Build history of the part. All positions in model axes, mm. A direction names the side the tool comes from. Give positions to 0.01 mm unless a question says otherwise; leave off trailing zeros. Write each loop counter-clockwise with the first axis right and the second up, starting at its lowest first coordinate (ties: lowest second). Pieces come first, ordered by that corner, then holes. Notation, with made-up numbers: (23.5, 34) -> (44.5, 34) arc R18 cw to (44.5, 51) -> close; hole circle Ø2 at (49.5, 9.5). An arc over 180 degrees is marked (long way). Put each result on its own line as item: value. Start each with the question number.
Item 1: Slice it at C-C, the plane x = 13. List the corners of the cut face in (y, z).
Item 2: Flat gauge pins, fed straight in: pin 1 Ø0.5 at (x, z) = (-16.5, 4.5) entering from -Y; pin 2 Ø3 at (y, z) = (-13.5, 5) entering from -X; pin 3 Ø0.7 at (x, z) = (-16.5, 3) entering from +Y; pin 4 Ø1.8 at (x, y) = (13, -5) entering from +Z. Where does each tip first touch, or does it go through?
Item 3: Slice it at B-B, the plane z = 5.5. List the corners of the cut face in (x, y).
Item 4: Tool access for faces 5 (the flat face through (0, 0, 4.2)), 6 (the flat face through (15.321, -9.837, 1.232)), 7 (the flat face through (-16.45, 7.76, 8.73)): list every direction of +Z, -Z, +X, -X, +Y, -Y with a clear straight run to the whole face (end or side of a thin tool).
Item 5: Slice it at A-A, the plane y = -5. List the corners of the cut face in (x, z).
Item 6: Drill centre lines: line 1 along X through (y, z) = (-5, 6.25); line 2 along Y through (x, z) = (-13, 5.5); line 3 along Z through (x, y) = (-16, -9.5). Where is each one in solid material? Low to high.
Item 7: Slice it at D-D, the plane x = 5. List the corners of the cut face in (y, z).
Item 8: Two-plate mould, pull along Z, no slides. Class faces 1 (the cylindrical face through (0.037, 3.795, 2.071)), 2 (the flat face through (0, 0, 10)), 3 (the flat face through (-2, -18, 2.5)), 4 (the flat face through (0, -4, 0)): pulls with the +Z half, pulls with the -Z half, needs draft (parallel to the pull), parting line crosses it, or undercut.
```python
from build123d import *

# Parameters (mm, degrees)
CROQUIS1_R                   = 17.7
SALIENTE_EXTRUIR1_DEPTH      = 10
ENVOLVER1_SECTION_W          = 1
ENVOLVER1_SECTION_H          = 2.5
ENVOLVER1_ANGLE              = 122.036773313
ENVOLVER1_SECTOR_2_SECTION_W = 1
ENVOLVER1_SECTOR_2_SECTION_H = 2.5
ENVOLVER1_SECTOR_2_ANGLE     = 122.036773313
SIMETR_A1_DEPTH              = 2.5
SIMETR_A1_START              = 7.5
SIMETR_A1_2_DEPTH            = 2.5
CAVIDAD1_DEPTH               = 4.2
SALIENTE_EXTRUIR2_START      = 4.2
SALIENTE_EXTRUIR2_DEPTH      = 4.2
CROQUIS6_R                   = 1.5
CORTAR_EXTRUIR1_DEPTH        = 10
CROQUIS8_W                   = 1.5
CROQUIS8_H                   = 1
CORTAR_EXTRUIR2_DEPTH        = 10
SIMETR_A4_COPY_1_SKETCH_R    = 1.5
SIMETR_A4_COPY_1_DEPTH       = 10
SIMETR_A4_COPY_2_SKETCH_W    = 1.5
SIMETR_A4_COPY_2_SKETCH_H    = 1
SIMETR_A4_COPY_2_DEPTH       = 10


# Read off the part's stored shape, not the designer's step: Simetría1, Cavidad1
with BuildPart() as part:
    # Croquis1 → Saliente-Extruir1 (new body)
    with BuildSketch(Plane.XY):
        Circle(CROQUIS1_R)
    extrude(amount=SALIENTE_EXTRUIR1_DEPTH)

    # Envolver1 section (on wrap section) → Envolver1 (revolve)
    with BuildSketch(Plane(origin=(0, 0, 0), x_dir=(-0.9043880828615337, 0.4267109039830592, 0), z_dir=(-0.4267109039830592, -0.9043880828615337, 0))):
        with Locations((18.2, -8.75)):
            Rectangle(ENVOLVER1_SECTION_W, ENVOLVER1_SECTION_H)
    revolve(axis=Axis((0, 0, 0), (0, 0, -1)), revolution_arc=ENVOLVER1_ANGLE)

    # Envolver1 sector 2 section (on wrap section) → Envolver1 sector 2 (revolve)
    with BuildSketch(Plane(origin=(0, 0, 0), x_dir=(-0.9043880828615337, 0.4267109039830592, 0), z_dir=(-0.4267109039830592, -0.9043880828615337, 0))):
        with Locations((18.2, -1.25)):
            Rectangle(ENVOLVER1_SECTOR_2_SECTION_W, ENVOLVER1_SECTOR_2_SECTION_H)
    revolve(axis=Axis((0, 0, 0), (0, 0, -1)), revolution_arc=ENVOLVER1_SECTOR_2_ANGLE)

    # Simetría1 outline → Simetría1 (add)
    with BuildSketch(Plane.XY):
        with BuildLine():
            ThreePointArc((-16.91205715, -7.979493904), (-1.214117133, -18.660544461), (15.735507416, -10.10365312))
            Line((15.735507416, -10.10365312), (14.894036431, -9.563350814))
            ThreePointArc((14.894036431, -9.563350814), (-1.149191083, -17.662654383), (-16.007669067, -7.552783))
            Line((-16.007669067, -7.552783), (-16.91205715, -7.979493904))
        make_face()
    extrude(amount=SIMETR_A1_DEPTH)

    # Simetr_a1 2 outline → Simetr_a1 2 (add)
    with BuildSketch(Plane.XY.offset(SIMETR_A1_START)):
        with BuildLine():
            ThreePointArc((-16.91205715, -7.979493904), (-1.214117133, -18.660544461), (15.735507416, -10.10365312))
            Line((15.735507416, -10.10365312), (14.894036431, -9.563350814))
            ThreePointArc((14.894036431, -9.563350814), (-1.149191083, -17.662654383), (-16.007669067, -7.552783))
            Line((-16.007669067, -7.552783), (-16.91205715, -7.979493904))
        make_face()
    extrude(amount=SIMETR_A1_2_DEPTH)

    # Cavidad1 outline → Cavidad1 (cut)
    with BuildSketch(Plane.XY):
        with BuildLine():
            Line((15.575034164, 2.196722968), (2.429979424, 2.915))
            ThreePointArc((2.429979424, 2.915), (0, 3.795), (-2.429979424, 2.915))
            Line((-2.429979424, 2.915), (-15.575034164, 2.196722968))
            ThreePointArc((-15.575034164, 2.196722968), (-17.655, 0), (-15.575034164, -2.196722968))
            Line((-15.575034164, -2.196722968), (-2.429979424, -2.915))
            ThreePointArc((-2.429979424, -2.915), (0, -3.795), (2.429979424, -2.915))
            Line((2.429979424, -2.915), (15.575034164, -2.196722968))
            ThreePointArc((15.575034164, -2.196722968), (17.655, 0), (15.575034164, 2.196722968))
        make_face()
    extrude(amount=CAVIDAD1_DEPTH, mode=Mode.SUBTRACT)

    # Croquis5 → Saliente-Extruir2 (add)
    with BuildSketch(Plane(origin=(0, 0, 4.2), x_dir=(-1, 0, 0), z_dir=(0, 0, -1)).offset(SALIENTE_EXTRUIR2_START)):
        with BuildLine():
            Line((16.6, -1.878556627), (16.6, 1.878556627))
            ThreePointArc((16.6, 1.878556627), (17.655, 0), (16.6, -1.878556627))
        make_face()
    saliente_extruir2 = extrude(amount=-SALIENTE_EXTRUIR2_DEPTH)

    # Simetría2: Saliente-Extruir2 across plane
    add(saliente_extruir2.mirror(Plane(origin=(0, 0, 0), x_dir=(0, 0, 1), z_dir=(1, 0, 0))))

    # Croquis6 → Cortar-Extruir1 (cut)
    with BuildSketch(Plane(origin=(0, 0, 0), x_dir=(-1, 0, 0), z_dir=(0, 0, -1))):
        with Locations((-13, 5)):
            Circle(CROQUIS6_R)
    cortar_extruir1 = extrude(amount=-CORTAR_EXTRUIR1_DEPTH, mode=Mode.SUBTRACT)

    # Croquis8 → Cortar-Extruir2 (cut)
    with BuildSketch(Plane(origin=(0, 0, 0), x_dir=(-1, 0, 0), z_dir=(0, 0, -1))):
        with Locations((-16.979104806, 5)):
            Rectangle(CROQUIS8_W, CROQUIS8_H)
    cortar_extruir2 = extrude(amount=-CORTAR_EXTRUIR2_DEPTH, mode=Mode.SUBTRACT)

    # Simetría3: Cortar-Extruir1, Cortar-Extruir2 across plane
    add(cortar_extruir1.mirror(Plane.ZX), mode=Mode.SUBTRACT)
    add(cortar_extruir2.mirror(Plane.ZX), mode=Mode.SUBTRACT)

    # Simetría4: Cortar-Extruir1, Cortar-Extruir2 across plane
    add(cortar_extruir1.mirror(Plane(origin=(0, 0, 0), x_dir=(0, 0, 1), z_dir=(1, 0, 0))), mode=Mode.SUBTRACT)
    add(cortar_extruir2.mirror(Plane(origin=(0, 0, 0), x_dir=(0, 0, 1), z_dir=(1, 0, 0))), mode=Mode.SUBTRACT)

    # Simetría4 copy 1 sketch → Simetría4 copy 1 (cut)
    with BuildSketch(Plane(origin=(0, 0, 0), x_dir=(1, 0, 0), z_dir=(0, 0, -1))):
        with Locations((-13, 5)):
            Circle(SIMETR_A4_COPY_1_SKETCH_R)
    extrude(amount=-SIMETR_A4_COPY_1_DEPTH, mode=Mode.SUBTRACT)

    # Simetría4 copy 2 sketch → Simetría4 copy 2 (cut)
    with BuildSketch(Plane(origin=(0, 0, 0), x_dir=(1, 0, 0), z_dir=(0, 0, -1))):
        with Locations((-16.979104806, 5)):
            Rectangle(SIMETR_A4_COPY_2_SKETCH_W, SIMETR_A4_COPY_2_SKETCH_H)
    extrude(amount=-SIMETR_A4_COPY_2_DEPTH, mode=Mode.SUBTRACT)


solid = part.part
```
Values follow:
1. outline: (-13.44, 0) -> (-6.5, 0) -> (-6.5, 10) -> (-13.44, 10) -> (-13.44, 7.5) -> (-12.01, 7.5) -> (-12.01, 2.5) -> (-13.44, 2.5) -> close; (-3.5, 0) -> (-2.34, 0) -> (-2.34, 4.2) -> (2.34, 4.2) -> (2.34, 0) -> (3.5, 0) -> (3.5, 10) -> (-3.5, 10) -> close; (6.5, 0) -> (13.44, 0) -> (13.44, 2.5) -> (12.01, 2.5) -> (12.01, 7.5) -> (13.44, 7.5) -> (13.44, 10) -> (6.5, 10) -> close
2. pin 1: y = -7.02
2. pin 2: x = -13.01
2. pin 3: y = 7.24
2. pin 4: through
3. outline: (-17.12, -4.5) -> (-16.23, -4.5) -> (-16.23, -5.5) -> (-16.82, -5.5) arc R17.7 ccw to (16.82, -5.5) -> (16.23, -5.5) -> (16.23, -4.5) -> (17.12, -4.5) arc R17.7 ccw to (17.12, 4.5) -> (16.23, 4.5) -> (16.23, 5.5) -> (16.82, 5.5) arc R17.7 ccw to (-16.82, 5.5) -> (-16.23, 5.5) -> (-16.23, 4.5) -> (-17.12, 4.5) arc R17.7 ccw to start; hole circle Ø3 at (-13, -5); hole circle Ø3 at (-13, 5); hole circle Ø3 at (13, -5); hole circle Ø3 at (13, 5)
4. face 5: -Z
4. face 6: +Z, -Z, +X
4. face 7: +Z, -Z, -X
5. outline: (-16.23, 0) -> (-14.5, 0) -> (-14.5, 10) -> (-16.23, 10) -> close; (-11.5, 0) -> (11.5, 0) -> (11.5, 10) -> (-11.5, 10) -> close; (14.5, 0) -> (16.23, 0) -> (16.23, 10) -> (14.5, 10) -> close
6. line 1: -16.23 to -14.5, -11.5 to 11.5, 14.5 to 16.23
6. line 2: -12.01 to -6.5, -3.5 to 3.5, 6.5 to 12.01
6. line 3: 0 to 2.5, 7.5 to 10
7. outline: (-18.02, 0) -> (-2.77, 0) -> (-2.77, 4.2) -> (2.77, 4.2) -> (2.77, 0) -> (18.02, 0) -> (18.02, 2.5) -> (16.98, 2.5) -> (16.98, 7.5) -> (18.02, 7.5) -> (18.02, 10) -> (-18.02, 10) -> (-18.02, 7.5) -> (-16.98, 7.5) -> (-16.98, 2.5) -> (-18.02, 2.5) -> close
8. face 1: needs draft
8. face 2: pulls with the +Z half
8. face 3: undercut
8. face 4: pulls with the -Z half
